For this review, use the dimensioned drawing (mm, ordinates from the lowest corner) and the shaded views. A direction names the side the tool comes from. Coordinates: 2 decimals unless noted, no trailing zeros. Write each loop counter-clockwise with the first axis right and the second up, starting at its lowest first coordinate (ties: lowest second). Pieces come first, ordered by that corner, then holes. Notation, with made-up numbers: (61.25, 49.5) - (98.25, 49.5) arc R26 ccw to (98.25, 84.5) - close; hole circle Ø5 at (11, 27). An arc over 180 degrees is marked (long way). Use one line per item in the form item = value. Start each with the question number.
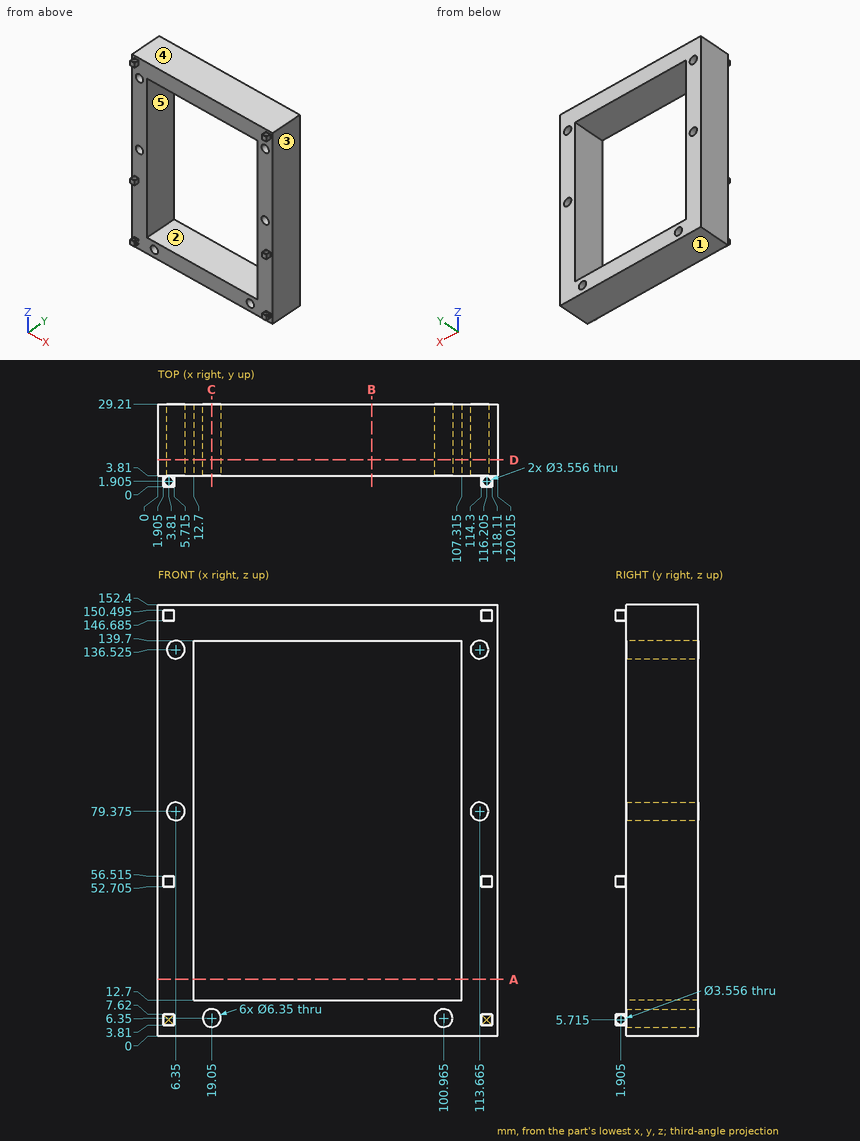
1. Take a section at C-C (x = 19.05). State the section outline as (y, z) points (3 decimals).
2. Take a section at D-D (y = 9.5). State the section outline as (x, z) points (3 decimals).
3. For the marked faces 4 and 5, list the 3-axis set-ups (+Z, -Z, +X, -X, +Y, -Y) from which the entire face can be reached by the end or side of a thin tool; tool diameter is ignored.
4. The part is to be moulded in two halves that separate along X. For the marked faces 1, 2 and 3, say which applies: released by +X, released by -X, zero draft, split by the parting line, or undercut.
5. Take a section at B-B (x = 75.5). State the section outline as (y, z) points.
6. For P1, Ø4, axis at y = 1, z = 5, coming from the +X side; P2, Ø4, axis at y = 3, z = 54, coming from the +X side (3 decimals); P3, Ø7.5, axis at x = 6.35, z = 136.525, coming from the -Y side; P4, Ø4, axis at y = 1.5, z = 5.5, coming from the -X side (3 decimals), all flat-tipped, find the tip position at first contact; note any pin that passes through.
7. Take a section at A-A (z = 20). State the section outline as (x, y) points (3 decimals), plus the area to 3 significant figures.
8. For L1, parallel to Z at x = 114, y = 4.25; L2, parallel to Z at x = 36.5, y = 8.25; L3, parallel to X at y = 16, z = 56.5 (3 decimals), list the stretches that pass through material, from the lowest coordinate up.
Returned:
q1.outline = (3.81, 0) - (29.21, 0) - (29.21, 3.175) - (3.81, 3.175) - close; (3.81, 9.525) - (29.21, 9.525) - (29.21, 12.7) - (3.81, 12.7) - close; (3.81, 139.7) - (29.21, 139.7) - (29.21, 152.4) - (3.81, 152.4) - close
q2.outline = (0, 0) - (120.015, 0) - (120.015, 152.4) - (0, 152.4) - close; hole circle Ø6.35 at (6.35, 79.375); hole circle Ø6.35 at (6.35, 136.525); hole (12.7, 12.7) - (107.315, 12.7) - (107.315, 139.7) - (12.7, 139.7) - close; hole circle Ø6.35 at (19.05, 6.35); hole circle Ø6.35 at (100.965, 6.35); hole circle Ø6.35 at (113.665, 79.375); hole circle Ø6.35 at (113.665, 136.525)
q3.face_4 = +Z, +X, -X, +Y, -Y
q3.face_5 = +Y, -Y
q4.face_1 = zero draft
q4.face_2 = undercut
q4.face_3 = released by +X
q5.outline = (3.81, 0) - (29.21, 0) - (29.21, 12.7) - (3.81, 12.7) - close; (3.81, 139.7) - (29.21, 139.7) - (29.21, 152.4) - (3.81, 152.4) - close
q6.P1 = 118.11
q6.P2 = 120.015
q6.P3 = 3.81
q6.P4 = 1.905
q7.outline = (0, 3.81) - (12.7, 3.81) - (12.7, 29.21) - (0, 29.21) - close; (107.315, 3.81) - (120.015, 3.81) - (120.015, 29.21) - (107.315, 29.21) - close
q7.area = 645 mm²
q8.L1 = 0 to 76.22, 82.53 to 133.37, 139.68 to 152.4
q8.L2 = 0 to 12.7, 139.7 to 152.4
q8.L3 = 0 to 12.7, 107.315 to 120.015
